```python
from build123d import *

# Parameters (mm, degrees)
SKETCH_1_R          = 1.5
SKETCH_1_R_2        = 7
EXTRUDE_1_DEPTH     = 2.25
SKETCH_5_W          = 13
SKETCH_5_H          = 28
EXTRUDE_3_DEPTH     = 3
SKETCH_6_R          = 1.5
CUT_EXTRUDE_2_DEPTH = 177.455253939
SKETCH_7_W          = 0.998721622
SKETCH_7_H          = 4.998741363
EXTRUDE_4_DEPTH     = 4.5
FILLET_1_R          = 10
CHAMFER_1_SIZE      = 3.5


with BuildPart() as part:
    # 草图1 → 凸台-拉伸1 (new, symmetric)
    with BuildSketch(Plane(origin=(0, 0, 0), x_dir=(0, 0, -1), z_dir=(1, 0, 0))):
        with BuildLine():
            ThreePointArc((97.745383074, -10), (109.768953128, -14.033657178), (116.949426552, -24.487241658))
            Line((116.949426552, -24.487241658), (130, -70))
            Line((130, -70), (150.805988717, -70))
            Line((150.805988717, -70), (132.020510773, -4.487252884))
            ThreePointArc((132.020510773, -4.487252884), (124.831577318, 5.972710201), (112.795276854, 10))
            Line((112.795276854, 10), (16, 10))
            ThreePointArc((16, 10), (11.149287499, 10.597149997), (6.588235294, 12.352941176))
            ThreePointArc((6.588235294, 12.352941176), (3.395498751, 13.581995002), (0, 14))
            Line((0, 14), (-18, 14))
            Line((-18, 14), (-18, 11))
            Line((-18, 11), (-13.388941598, -4.090995342))
            ThreePointArc((-13.388941598, -4.090995342), (-8.328447191, -11.253309175), (0, -14))
            Line((0, -14), (13.224243357, -14))
            Line((13.224243357, -14), (13.224243357, -10.193557234))
            ThreePointArc((13.224243357, -10.193557234), (14.608751519, -10.048447989), (16, -10))
            Line((16, -10), (97.745383074, -10))
        make_face()
        with Locations((138.148241349, -62.136741787)):
            Circle(SKETCH_1_R, mode=Mode.SUBTRACT)
        with Locations((129.879120675, -33.298890909)):
            Circle(SKETCH_1_R, mode=Mode.SUBTRACT)
        with Locations((0, -10.5)):
            Circle(SKETCH_1_R, mode=Mode.SUBTRACT)
        with Locations((-10.5, 0)):
            Circle(SKETCH_1_R, mode=Mode.SUBTRACT)
        Circle(SKETCH_1_R_2, mode=Mode.SUBTRACT)
        with Locations((10.5, 0)):
            Circle(SKETCH_1_R, mode=Mode.SUBTRACT)
        with Locations((0, 10.5)):
            Circle(SKETCH_1_R, mode=Mode.SUBTRACT)
        with Locations((40.5, 0)):
            Circle(SKETCH_1_R, mode=Mode.SUBTRACT)
        with Locations((70.5, 0)):
            Circle(SKETCH_1_R, mode=Mode.SUBTRACT)
        with Locations((100.5, 0)):
            Circle(SKETCH_1_R, mode=Mode.SUBTRACT)
        with Locations((121.61, -4.461040031)):
            Circle(SKETCH_1_R, mode=Mode.SUBTRACT)
    extrude(amount=EXTRUDE_1_DEPTH, both=True)

    # 草图5 → 凸台-拉伸3 (add)
    with BuildSketch(Plane.XZ.offset(70)):
        with Locations((4.25, -140.805988717)):
            Rectangle(SKETCH_5_W, SKETCH_5_H)
    extrude(amount=EXTRUDE_3_DEPTH)

    # 草图6 → 切除-拉伸2 (cut, through all)
    with BuildSketch(Plane(origin=(0, -70, 0), x_dir=(1, 0, 0), z_dir=(0, 1, 0))):
        with Locations(Location((6.25, 149.805988717, 0), (0, 0, 270))):
            Circle(SKETCH_6_R)
        with Locations(Location((6.25, 131.805988717, 0), (0, 0, 90))):
            Circle(SKETCH_6_R)
    extrude(amount=-CUT_EXTRUDE_2_DEPTH, mode=Mode.SUBTRACT)

    # 草图7 → 凸台-拉伸4 (add)
    with BuildSketch(Plane(origin=(2.25, 0, 0), x_dir=(0, 0, -1), z_dir=(1, 0, 0))):
        with Locations((-16.501706932, 16.499370682)):
            Rectangle(SKETCH_7_W, SKETCH_7_H)
    extrude(amount=-EXTRUDE_4_DEPTH)

    # 圆角1
    # the kernel refuses this fillet: 10 mm, written as the material it adds along each edge
    with BuildSketch(Plane(origin=(2.25, 14, 16.002346121), x_dir=(0, 0, -1), z_dir=(-1, 0, 0))) as fillet_1_piece_1:
        with BuildLine():
            CenterArc((8.659527241, -10), FILLET_1_R, 90, 59.991672573)
            Line((0, -4.998741363), (-0.173190545, -4.89871619))
            ThreePointArc((-0.173190545, -4.89871619), (-0.2, -2.499370681), (-0.2, 0))
            Line((-0.2, 0), (0, 0.2))
            Line((0, 0.2), (8.659527241, 0.2))
            Line((8.659527241, 0.2), (8.659527241, 0))
        make_face()
    extrude(amount=4.5)
    with BuildSketch(Plane(origin=(2.25, 14, 17.001067743), x_dir=(0, 0, 1), z_dir=(-1, 0, 0))) as fillet_1_piece_2:
        with BuildLine():
            CenterArc((10, 4.356693642), FILLET_1_R, 180, 25.82789421)
            Line((0, 4.356693642), (-0.2, 4.356693642))
            Line((-0.2, 4.356693642), (-0.2, 0))
            Line((-0.2, 0), (0, -0.2))
            ThreePointArc((0, -0.2), (0.499466129, -0.2), (0.818910902, -0.087133873))
            Line((0.818910902, -0.087133873), (0.998932257, 0))
        make_face()
    extrude(amount=4.5)

    # 倒角1
    chamfer_1_edges = [part.edges().sort_by_distance(p)[0] for p in [
        (10.75, -71.5, -154.805988717),
        (10.75, -71.5, -126.805988717),
    ]]
    chamfer(chamfer_1_edges, length=CHAMFER_1_SIZE)


solid = part.part
```
Input: part model. Units: mm. Frame: model coordinates. A direction names the side the tool comes from. Give positions to 0.01 mm unless a question says otherwise; leave off trailing zeros. Loops run counter-clockwise (first coordinate to the right, second up) from the corner with the lowest first, then second, coordinate; pieces in that order, holes last. Notation, with made-up numbers: M 33.5,-8.75 L 56.5,-8.75 A21 ccw 56.5,11.25 Z; hole C 9,7 d3. An arc over 180 degrees is marked long. Answer as CSV lines item,"result". Start each with the question number.
1. Line query: L1, parallel to Y at x = 0.3, z = 0; L2, parallel to Y at x = 4, z = -145.5; L3, parallel to Y at x = 0.25, z = -10.5. Output: solid intervals per line, ascending.
2. Section B-B on x = -0.5. State how many separate pieces and enclosed holes the cut face has, plus the area to 3 significant figures.
3. Section C-C on y = -44. Return loops of the section in (x, z).
4. Section A-A on z = -47.5. Return loops of the section in (x, y).
5. Reachability of faces 4 (the face through (2.25, -9, -79)), 5 (the face through (0.031, -46.925, -123.383)), 6 (the face through (2, -71, -126.806)), 7 (the face through (0, 9, 0)), 8 (the face through (0, -12, -13.224)) from +Z, -Z, +X, -X, +Y, -Y: full face, straight path, thin tool, end or side. Return the list, or none.
6. Pin query (flat end, axial travel): P1, Ø5, axis at x = 2.5, z = -43.5, coming from the -Y side; P2, Ø2, axis at x = 0.5, z = 5, coming from the +Y side; P3, Ø5, axis at y = 0, z = -100.5, coming from the +X side. Return the tip coordinate at first contact, or that it passes through.
7. Pull-direction query (Y, two-part tool) for faces 1 (the face through (0, -12, 0)), 2 (the face through (0.03, 10.58, -11.22)), 3 (the face through (0, 13, 18)); classes: released by +Y, released by -Y, zero draft, split by the parting line, or undercut.
Computed values:
1,L1,"y = -14 to -12, -9 to -7, 7 to 9, 12 to 14"
1,L2,"y = -73 to -70"
1,L3,"y = -14 to -1.5, 1.5 to 10.77"
2,separate pieces,"1"
2,enclosed holes,"11"
2,area,"4,210 mm²"
3,outline,"M -2.25,-143.35 L 2.25,-143.35 L 2.25,-122.54 L -2.25,-122.54 Z"
4,outline,"M -2.25,-10 L 2.25,-10 L 2.25,10 L -2.25,10 Z"
5,face 4,"+Z, -Z, +X, +Y"
5,face 5,"+Z, +X, -X"
5,face 6,"+Z, +X, -X, -Y"
5,face 7,"+X, -X"
5,face 8,"+X, -X, -Y"
6,P1,"stops at y = -10"
6,P2,"stops at y = 14"
6,P3,"stops at x = 2.25"
7,face 1,"undercut"
7,face 2,"released by +Y"
7,face 3,"zero draft"
